The listing builds one solid part. Answer for the finished solid, in the listing's coordinates (mm). A direction names the side the tool comes from. Round coordinates to 2 decimals unless told otherwise and drop trailing zeros. Loops run counter-clockwise (first coordinate to the right, second up) from the corner with the lowest first, then second, coordinate; pieces in that order, holes last. Notation, with made-up numbers: M 19,-4 L 46,-4 A22 cw 46,20 Z; hole C 22,13 d7. An arc over 180 degrees is marked long. Answer as a JSON object with one key per item and string values.
```python
from build123d import *

# Parameters (mm, degrees)
F0_W     = 177.861019969
F0_H     = 164.4679009914
F1_DEPTH = 6.35
F2_W     = 59.2979416251
F2_H     = 61.2313710153
F3_DEPTH = 76.2
F4_W     = 47.6095601916
F4_H     = 47.6991081774
F5_DEPTH = 38.1
F6_W     = 24.9475054443
F6_H     = 37.8527449608
F7_DEPTH = 38.1


with BuildPart() as f1:
    # F0 (on Top) → F1 (new body)
    with BuildSketch(Plane.XY):
        with Locations((-0.550635159, -1.3211369514)):
            Rectangle(F0_W, F0_H)
    extrude(amount=F1_DEPTH)

    # F2 (on face) → F3 (join)
    with BuildSketch(Plane.XY.offset(6.35)):
        with Locations((2.9982812703, -3.9570573717)):
            Rectangle(F2_W, F2_H)
    extrude(amount=F3_DEPTH)

    # F4 (on face) → F5 (join)
    with BuildSketch(Plane.XZ.offset(34.5727428794)):
        with Locations((-2.8459094465, 30.1995540887)):
            Rectangle(F4_W, F4_H)
    extrude(amount=F5_DEPTH)

    # F6 (on face) → F7 (cut)
    with BuildSketch(Plane.YZ.offset(20.9588706493)):
        with Locations((-53.0296508223, 25.2763724804)):
            Rectangle(F6_W, F6_H)
    extrude(amount=-F7_DEPTH, mode=Mode.SUBTRACT)


solid = f1.part
```
Item 1: Flat-ended cylindrical pins translate along their axes: P1, Ø3, axis at y = -7.5, z = 65, coming from the -X side; P2, Ø24, axis at x = 7.5, z = 32.5, coming from the -Y side; P3, Ø3, axis at x = 22.5, y = -62, coming from the +Z side. Find the tip coordinate at first contact, or state that the pin passes through.
Values follow:
{"P1": "x = -26.65", "P2": "y = -72.67", "P3": "z = 6.35"}
Item 2: Which of the six approach directions +Z, -Z, +X, -X, +Y, -Y give full straight-line access (tool end or side, diameter ignored) to faces 1 (the face through (32.647, -4, 44)), 2 (the face through (-3, -72.673, 31)), 3 (the face through (-17.141, -53, 26))?
Values follow:
{"face 1": "+Z, +X, +Y, -Y", "face 2": "+Z, +X, -X, -Y", "face 3": "+X"}
Item 3: The part is cut by section A-A (x = 15.5). Give the vertices of the cut face in (y, z).
Values follow:
{"outline": "M -83.56,0 L 80.91,0 L 80.91,6.35 L 26.66,6.35 L 26.66,82.55 L -34.57,82.55 L -34.57,54.05 L -72.67,54.05 L -72.67,6.35 L -83.56,6.35 Z; hole M -65.5,6.35 L -40.56,6.35 L -40.56,44.2 L -65.5,44.2 Z"}
Item 4: The part is cut by section B-B (z = 17). Give the vertices of the cut face in (x, y), then the cut area to 3 significant figures.
Values follow:
{"outline": "M -26.65,-72.67 L 20.96,-72.67 L 20.96,-65.5 L -17.14,-65.5 L -17.14,-40.56 L 20.96,-40.56 L 20.96,-34.57 L 32.65,-34.57 L 32.65,26.66 L -26.65,26.66 Z", "area": "4,490 mm^2"}
Item 5: The part is cut by section C-C (y = -61). Give the vertices of the cut face in (x, z), then the cut area to 3 significant figures.
Values follow:
{"outline": "M -89.48,0 L 88.38,0 L 88.38,6.35 L -17.14,6.35 L -17.14,44.2 L 20.96,44.2 L 20.96,54.05 L -26.65,54.05 L -26.65,6.35 L -89.48,6.35 Z", "area": "1,960 mm^2"}
Item 6: Determine the mould class of faces 4 (the face through (3, 26.659, 44)), 5 (the face through (2, -53, 44.203)), 6 (the face through (-26.651, -22, 44)), 7 (the face through (2, -40.556, 25)) for opening direction Y: released by +Y, released by -Y, zero draft, split by the parting line, or undercut.
Values follow:
{"face 4": "released by +Y", "face 5": "undercut", "face 6": "zero draft", "face 7": "undercut"}
Item 7: Straight lines are drawn through the part: line 1 (Y direction, x = -8, z = 9.5); line 2 (Y direction, x = -20, z = 19); line 3 (Z direction, x = -44.5, y = -38). For each, find the intervals that lie inside material, in ascending order.
Values follow:
{"line 1": "-72.67 to -65.5, -40.56 to 26.66", "line 2": "-72.67 to 26.66", "line 3": "0 to 6.35"}
Item 8: The part is cut by section D-D (x = -42.5). Give the vertices of the cut face in (y, z).
Values follow:
{"outline": "M -83.56,0 L 80.91,0 L 80.91,6.35 L -83.56,6.35 Z"}
